Can you work these out from the model? Positions are in its coordinate system, mm. Round coordinates to 2 decimals unless told otherwise and drop trailing zeros. Order: outer loops, then holes, each group sorted by start corner. A loop starts at its lowest first (then second) coordinate and runs counter-clockwise, first axis right, second up. Notation, with made-up numbers: M 51,84.5 L 79,84.5 A21 ccw 79,97.5 Z; hole C 12,55 d7. An arc over 180 degrees is marked long. Answer as CSV lines item,"result". Start each with the question number.
Autodesk Inventor part; units mm, degrees
ref_plane "YZ Plane" through (0, 0, 0) normal (1, 0, 0) x (0, 1, 0)
ref_plane "XZ Plane" through (0, 0, 0) normal (0, 1, 0) x (-1, 0, 0)
ref_plane "XY Plane" through (0, 0, 0) normal (0, 0, 1) x (1, 0, 0)
sketch "Skizze1" plane through (0, 0, 0) normal (0, 0, 1) x (1, 0, 0)
  circle A0 centre (2.5, 77) radius 1.875 construction
  circle A1 centre (45.5, 77) radius 1.875 construction
  circle A2 centre (2.5, 8) radius 1.875 construction
  circle A3 centre (45.5, 8) radius 1.875 construction
  line L0 (-1, 5) -> (-1, 80) construction
  line L1 (49, 5) -> (-1, 5) construction
  line L2 (49, 80) -> (49, 5) construction
  line L3 (-1, 80) -> (49, 80) construction
  circle A4 centre (63.5, 77) radius 1.875 construction
  circle A5 centre (106.5, 77) radius 1.875 construction
  circle A6 centre (63.5, 8) radius 1.875 construction
  circle A7 centre (106.5, 8) radius 1.875 construction
  line L4 (60, 5) -> (60, 80) construction
  line L5 (110, 5) -> (60, 5) construction
  line L6 (110, 80) -> (110, 5) construction
  line L7 (60, 80) -> (110, 80) construction
  line L8 (-3, 0) -> (-3, 85) construction
  line L9 (-23, 0) -> (-23, 85) construction
  line L10 (-16.375, 0) -> (-21, 0) construction
  line L11 (-23, 0) -> (-21, 0) construction
  line L12 (-16.375, 0) -> (-15.575, 0) construction
  line L13 (0, 0) -> (-9.625, 0) construction
  line L14 (118.625, 85) -> (114, 85) construction
  line L15 (114, 0) -> (114, 85) construction
  line L16 (118.625, 0) -> (114, 0) construction
  line L17 (118.625, 0) -> (118.625, 85) construction
  line L18 (112, 0) -> (114, 0) construction
  line L19 (112, 0) -> (112, 85) construction
  line L20 (132, 0) -> (132, 85) construction
  line L21 (130, 0) -> (132, 0) construction
  line L22 (-23, 0) -> (132, 0)
  line L23 (132, 0) -> (132, 5)
  line L24 (132, 5) -> (-23, 5)
  line L25 (-23, 5) -> (-23, 0)
  line L26 (102, 13) -> (132, 13)
  line L27 (132, 13) -> (132, 5)
  line L28 (132, 5) -> (102, 5)
  line L29 (102, 5) -> (102, 13)
  line L30 (41, 5) -> (68, 5)
  line L31 (68, 5) -> (68, 13)
  line L32 (68, 13) -> (41, 13)
  line L33 (41, 13) -> (41, 5)
  line L34 (-23, 5) -> (7, 5)
  line L35 (7, 5) -> (7, 13)
  line L36 (7, 13) -> (-23, 13)
  line L37 (-23, 13) -> (-23, 5)
  line L38 (49, 5) -> (60, 5) construction
  line L39 (54.5, 0.9478) -> (54.5, 9.0522) construction
  line L40 (130, 0) -> (114, 0) construction
  line L41 (114, 0) -> (114, 13) construction
  line L42 (114, 13) -> (130, 13) construction
  line L43 (130, 13) -> (130, 0) construction
  line L44 (130, 0) -> (114, 13) construction
  line L45 (114, 0) -> (130, 13) construction
  line L46 (-23, 0) -> (-3, 0) construction
  line L47 (-3, 0) -> (-3, 13) construction
  line L48 (-3, 13) -> (-23, 13) construction
  line L49 (-23, 13) -> (-23, 0) construction
  line L50 (-23, 0) -> (-3, 13) construction
  line L51 (-3, 0) -> (-23, 13) construction
  point P0 (54.5, 5)
  point P1 (122, 6.5)
  point P2 (-13, 6.5)
  dimension "d0" = 8
  dimension "d1" = 8
  dimension "d2" = 8
extrude "Extrusion1" add sketch "Skizze1" along normal blind 2
sketch "Skizze2" plane through (0, 0, 0) normal (0, 0, -1) x (-1, 0, 0)
  point P0 (0, 0)
  point P1 (-106.5, 8)
  point P2 (-63.5, 8)
  point P3 (-45.5, 8)
  point P4 (-2.5, 8)
hole "Bohrung1" at (106.5, 8, 0) at (63.5, 8, 0) at (45.5, 8, 0) at (2.5, 8, 0) direction (0, 0, 1) diameter 2.459 end through all
fillet "Rundung1" radius 2 12 edges at (102, 5, 1) (102, 13, 1) (68, 5, 1) (68, 13, 1) (41, 13, 1) (41, 5, 1) (7, 5, 1) (7, 13, 1) (-23, 13, 1) (-23, 0, 1) (132, 0, 1) (132, 13, 1)
sketch "Skizze3" plane through (0, 0, 0) normal (0, 0, -1) x (-1, 0, 0)
  point P0 (0, 0)
  point P1 (13, 6.5)
  point P2 (-122, 6.5)
hole "Bohrung2" at (-13, 6.5, 0) at (122, 6.5, 0) direction (0, 0, 1) diameter 4.2 end through all
properties part number "DriverMount" material "Aluminium 6061"
(1) If I drill on line 1 along Y through (x, z) = (45.5, 1.4); line 2 along Y through (x, z) = (122, 1.15); line 3 along X through (y, z) = (12, 1.75), over which ranges is the centre line in solid material (lowest first)?
(2) I want a section at B-B on x = -13. Write out the boundary of the cut face in (y, z), and give its area (3 significant figures).
(3) I want a section at C-C on x = 27. Write out the boundary of the cut face in (y, z).
(4) I'm going to push a flat-ended pin straight in: P1, Ø1, axis at x = 18.5, z = 1, coming from the +Y side. Where does the tip first touch, or does it pass through?
(5) I want a section at A-A on z = 0.55. Count the separate pieces of the cut face and the enclosed holes in it, and give its area (3 significant figures).
From the geometry:
1,line 1,"0 to 6.77, 9.23 to 13"
1,line 2,"0 to 4.4, 8.6 to 13"
1,line 3,"-22.73 to 6.73, 41.27 to 67.73, 102.27 to 131.73"
2,outline,"M 0,0 L 4.4,0 L 4.4,2 L 0,2 Z; M 8.6,0 L 13,0 L 13,2 L 8.6,2 Z"
2,area,"17.6 mm²"
3,outline,"M 0,0 L 5,0 L 5,2 L 0,2 Z"
4,P1,"y = 5"
5,separate pieces,"1"
5,enclosed holes,"6"
5,area,"1,420 mm²"
